from build123d import *

# Parameters (mm, degrees)
F0_W     = 50
F0_H     = 45
F1_DEPTH = 7
F3_D     = 4.2
F5_D     = 4.5
F7_D     = 2.5


with BuildPart() as f1:
    # F0 (on Top) → F1 (new body)
    with BuildSketch(Plane.XY):
        with Locations((15.1915311813, 4.4455631077)):
            Rectangle(F0_W, F0_H)
    extrude(amount=F1_DEPTH)

    # F3 (through all)
    with Locations(Plane.XY.offset(7)):
        with Locations((32.1915311813, 20.4455631077), (32.1915311813, -11.5544368923)):
            Hole(F3_D / 2)

    # F5 (through all)
    with Locations(Plane.XY.offset(7)):
        with Locations((-3.8084688187, 13.4455631077), (20.1915311813, 13.4455631077), (20.1915311813, -4.5544368923), (-3.8084688187, -4.5544368923)):
            Hole(F5_D / 2)

    # F7 (through all)
    with Locations(Plane(origin=(0, 0, 0), x_dir=(1, 0, 0), z_dir=(0, 0, -1))):
        with Locations((0.1915311813, 14.0544368923), (16.1915311813, 14.0544368923), (16.1915311813, -22.9455631077), (0.1915311813, -22.9455631077)):
            Hole(F7_D / 2)


solid = f1.part
Work out the finished part from the listing and answer in its coordinate system (mm). Give positions to 0.01 mm unless a question says otherwise; leave off trailing zeros. Order: outer loops, then holes, each group sorted by start corner. A loop starts at its lowest first (then second) coordinate and runs counter-clockwise, first axis right, second up. Notation, with made-up numbers: (-35, -30.75) - (14, -30.75) arc R18 ccw to (14, -24.75) - close; hole circle Ø6 at (89.25, 8). An arc over 180 degrees is marked (long way). Answer as CSV lines item,"result". Start each with the question number.
Q1. The part is cut by section A-A (y = 21). Write down the section's boundary in (x, z), then the cut area to 3 significant figures.
Q2. The mould has two halves that part along Y. Classify faces 1 (the face through (15, -18.054, 3)), 2 (the face through (15, 5, 0)), 3 (the face through (15, 26.946, 3)), 4 (the face through (18.045, -3.879, 3.451)): +Y half, -Y half, draft (parallel to the pull), parting line (faces both ways), or undercut.
Q3. Find the intervals of material crossed by L1, parallel to X at y = 23, z = 6.75; L2, parallel to Y at x = 17, z = 6.75; L3, parallel to Y at x = -4, z = 2.5, in increasing order. Write a range as [from, to].
Q4. The part is cut by section B-B (x = -2.5). Write down the section's boundary in (y, z), then the cut area to 3 significant figures.
Q5. The part is cut by section C-C (z = 0.75). Give the number of separate pieces and of enclosed holes in the cut face, then the cut area to 3 significant figures.
Check result:
1,outline,"(-9.81, 0) - (30.17, 0) - (30.17, 7) - (-9.81, 7) - close; (34.22, 0) - (40.19, 0) - (40.19, 7) - (34.22, 7) - close"
1,area,"322 mm²"
2,face 1,"-Y half"
2,face 2,"draft"
2,face 3,"+Y half"
2,face 4,"undercut"
3,L1,"x = [-9.81, -1.06], [1.44, 14.94], [17.44, 40.19]"
3,L2,"y = [-18.05, -15.01], [-13.1, 21.99], [23.9, 26.95]"
3,L3,"y = [-18.05, -6.8], [-2.31, 11.2], [15.69, 26.95]"
4,outline,"(-18.05, 0) - (-6.38, 0) - (-6.38, 7) - (-18.05, 7) - close; (-2.72, 0) - (11.62, 0) - (11.62, 7) - (-2.72, 7) - close; (15.28, 0) - (26.95, 0) - (26.95, 7) - (15.28, 7) - close"
4,area,"264 mm²"
5,separate pieces,"1"
5,enclosed holes,"10"
5,area,"2,140 mm²"
